For this review, take the finished solid that the model builds, in its own axes (mm). Round coordinates to 2 decimals unless told otherwise and drop trailing zeros. Put each result on its own line as item: value.
from build123d import *

# Parameters (mm, degrees)
SKETCH1_R           = 2
BOSS_EXTRUDE2_DEPTH = 1257.3
FILLET1_R           = 1.065
FILLET4_R           = 2.13
FILLET5_R           = 2.13
FILLET8_R           = 0.5325
FILLET11_R          = 0.5325
FILLET15_R          = 3
FILLET16_R          = 3


with BuildPart() as part:
    # Sketch1 → Boss-Extrude2 (new body)
    with BuildSketch(Plane.XY):
        Polygon((7.345, 3.97), (3.25, -1.87), (-3.25, -1.87), (-7.345, 3.97), (-3.25, 3.97), (-3.25, 6.25), (-12.5, 6.25), (-12.5, -6.25), (12.5, -6.25), (12.5, 6.25), (3.25, 6.25), (3.25, 3.97), align=None)
        with Locations((-8.5, -2.25)):
            Circle(SKETCH1_R, mode=Mode.SUBTRACT)
        with Locations((8.5, -2.25)):
            Circle(SKETCH1_R, mode=Mode.SUBTRACT)
    extrude(amount=BOSS_EXTRUDE2_DEPTH)

    # Fillet1
    fillet1_edges = [part.edges().sort_by_distance(p)[0] for p in [
        (3.25, 3.97, 628.65),
        (3.25, 6.25, 628.65),
        (-3.25, 6.25, 628.65),
        (-3.25, 3.97, 628.65),
    ]]
    fillet(fillet1_edges, radius=FILLET1_R)

    # Fillet4
    fillet4_edges = [part.edges().sort_by_distance(p)[0] for p in [
        (12.5, 6.25, 628.65),
    ]]
    fillet(fillet4_edges, radius=FILLET4_R)

    # Fillet5
    fillet5_edges = [part.edges().sort_by_distance(p)[0] for p in [
        (12.5, -6.25, 628.65),
        (-12.5, -6.25, 628.65),
        (-12.5, 6.25, 628.65),
    ]]
    fillet(fillet5_edges, radius=FILLET5_R)

    # Fillet8
    fillet8_edges = [part.edges().sort_by_distance(p)[0] for p in [
        (7.345, 3.97, 628.65),
    ]]
    fillet(fillet8_edges, radius=FILLET8_R)

    # Fillet11
    fillet11_edges = [part.edges().sort_by_distance(p)[0] for p in [
        (-7.345, 3.97, 628.65),
    ]]
    fillet(fillet11_edges, radius=FILLET11_R)

    # Fillet15
    fillet15_edges = [part.edges().sort_by_distance(p)[0] for p in [
        (-3.25, -1.87, 628.65),
    ]]
    fillet(fillet15_edges, radius=FILLET15_R)

    # Fillet16
    fillet16_edges = [part.edges().sort_by_distance(p)[0] for p in [
        (3.25, -1.87, 628.65),
    ]]
    fillet(fillet16_edges, radius=FILLET16_R)


solid = part.part
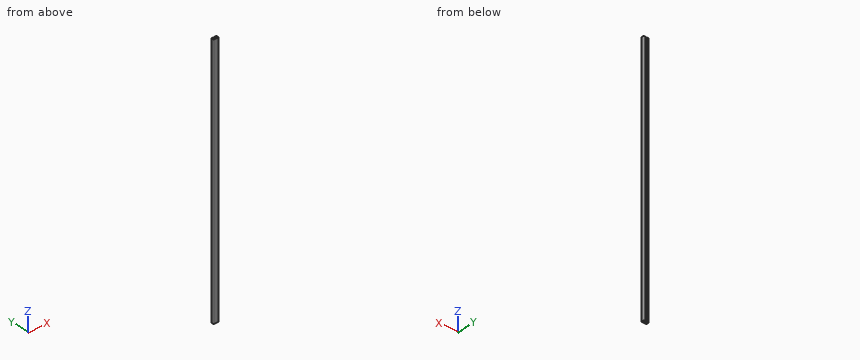
(1) To check wall thickness, follow L1, parallel to X at y = -1.5, z = 553; L2, parallel to X at y = -0.5, z = 572; L3, parallel to Y at x = -4.25, z = 873. State the ranges of each line that lie inside material, in increasing order.
A:
L1: x = -12.5 to -10.35, -6.65 to -3.13, 3.13 to 6.65, 10.35 to 12.5
L2: x = -12.5 to -9.47, -7.53 to -4.21, 4.21 to 7.53, 9.47 to 12.5
L3: y = -6.25 to -0.44, 3.97 to 6.25
(2) Insertion check: pin 1 Ø1 at (x, z) = (0, 553.5) entering from +Y. The pin has a flat end and moves straight along its axis. Give the tip position at first contact, or say it passes through.
A:
pin 1: stops at y = -1.87
(3) Add section A-A on z = 1092. State how many separate pieces and enclosed holes the cut face has, then the cut area to 3 significant figures.
A:
separate pieces: 1
enclosed holes: 2
area: 207 mm2
